```python
from build123d import *

# Parameters (mm, degrees)
CHAMFER1_SIZE = 0.5


with BuildPart() as part:
    # Sketch1 → Revolve1 (revolve)
    with BuildSketch(Plane.XY):
        with BuildLine():
            Line((1.75, 0), (1.75, 10.5))
            Line((1.75, 10.5), (3.9, 10.5))
            Line((3.9, 10.5), (3.9, 5.5))
            Line((3.9, 5.5), (4.9, 5.5))
            ThreePointArc((4.9, 5.5), (5.177696338, 2.695539268), (6, 0))
            Line((6, 0), (1.75, 0))
        make_face()
    revolve(axis=Axis((0, -1052.626814563, 0), (0, 1, 0)))

    # Chamfer1
    # the kernel refuses this chamfer: 0.5 mm, written as the material it takes off along each edge
    with BuildSketch(Plane(origin=(0, 0, 0), x_dir=(1, 0, 0), z_dir=(0, 0, 1))) as chamfer1_piece_1:
        Polygon((1.75 + CHAMFER1_SIZE, 0), (1.75, CHAMFER1_SIZE), (1.75, 0), align=None)
    revolve(axis=Axis((0, 0, 0), (0, 1, 0)), mode=Mode.SUBTRACT)
    with BuildSketch(Plane(origin=(0, 10.5, 0), x_dir=(1, 0, 0), z_dir=(0, 0, 1))) as chamfer1_piece_2:
        Polygon((1.75, -CHAMFER1_SIZE), (1.75 + CHAMFER1_SIZE, 0), (1.75, 0), align=None)
    revolve(axis=Axis((0, 10.5, 0), (0, 1, 0)), mode=Mode.SUBTRACT)
    with BuildSketch(Plane(origin=(0, 10.5, 0), x_dir=(1, 0, 0), z_dir=(0, 0, 1))) as chamfer1_piece_3:
        Polygon((3.9 - CHAMFER1_SIZE, 0), (3.9, -CHAMFER1_SIZE), (3.9, 0), align=None)
    revolve(axis=Axis((0, 10.5, 0), (0, 1, 0)), mode=Mode.SUBTRACT)
    with BuildSketch(Plane(origin=(0, 5.5, 0), x_dir=(1, 0, 0), z_dir=(0, 0, 1))) as chamfer1_piece_4:
        with BuildLine():
            Line((4.9 - CHAMFER1_SIZE, 0), (4.909063924, -0.509063924))
            ThreePointArc((4.909063924, -0.509063924), (4.902396158, -0.261771596), (4.9, 0))
            Line((4.9, 0), (4.9 - CHAMFER1_SIZE, 0))
        make_face()
    revolve(axis=Axis((0, 5.5, 0), (0, 1, 0)), mode=Mode.SUBTRACT)


solid = part.part
```
Read the model definition and answer for the solid it produces. Units are mm, in the model's axes. Coordinates: 2 decimals unless noted, no trailing zeros. Loops run counter-clockwise (first coordinate to the right, second up) from the corner with the lowest first, then second, coordinate; pieces in that order, holes last. Notation, with made-up numbers: (40, -5.75) - (51, -5.75) arc R32 ccw to (51, 24.25) - close; hole circle Ø11 at (55, 21). An arc over 180 degrees is marked (long way). Answer in a Markdown table with one row per item.
1. Determine the mould class of faces 1 (the face through (3, 0, 0)), 2 (the face through (-2.87, 7.72, -2.64)), 3 (the face through (1.617, 5.316, 0.67)) for opening direction X: +X half, -X half, draft (parallel to the pull), parting line (faces both ways), or undercut.
Conclusion:
| item | result |
|---|---|
| face 1 | draft |
| face 2 | parting line |
| face 3 | undercut |
2. Find section A-A, the plane x = 0. Write down the section's boundary in (y, z), then the cut area to 3 significant figures.
Conclusion:
| item | result |
|---|---|
| outline | (0, -6) arc R14.3 cw to (4.99, -4.91) - (5.5, -4.4) - (5.5, -3.9) - (10, -3.9) - (10.5, -3.4) - (10.5, -2.25) - (10, -1.75) - (0.5, -1.75) - (0, -2.25) - close; (0, 2.25) - (0.5, 1.75) - (10, 1.75) - (10.5, 2.25) - (10.5, 3.4) - (10, 3.9) - (5.5, 3.9) - (5.5, 4.4) - (4.99, 4.91) arc R14.3 cw to (0, 6) - close |
| area | 59.1 mm² |
3. Straight lines are drawn through the part: line 1 (Z direction, x = 0, y = 6.5); line 2 (X direction, y = 3, z = -0.5). For each, find the intervals that lie inside material, in ascending order.
Conclusion:
| item | result |
|---|---|
| line 1 | z = -3.9 to -1.75, 1.75 to 3.9 |
| line 2 | x = -5.1 to -1.68, 1.68 to 5.1 |
4. Find section B-B, the plane z = 0. Write down the section's boundary in (x, y), then the cut area to 3 significant figures.
Conclusion:
| item | result |
|---|---|
| outline | (-6, 0) - (-2.25, 0) - (-1.75, 0.5) - (-1.75, 10) - (-2.25, 10.5) - (-3.4, 10.5) - (-3.9, 10) - (-3.9, 5.5) - (-4.4, 5.5) - (-4.91, 4.99) arc R14.3 cw to start; (1.75, 0.5) - (2.25, 0) - (6, 0) arc R14.3 cw to (4.91, 4.99) - (4.4, 5.5) - (3.9, 5.5) - (3.9, 10) - (3.4, 10.5) - (2.25, 10.5) - (1.75, 10) - close |
| area | 59.1 mm² |
5. Given pin 1 (3 mm diameter, centred on x = 0, z = 0, fed in from +Y); pin 2 (4 mm diameter, centred on x = -0.5, z = -0.5, fed in from +Y); pin 3 (2 mm diameter, centred on y = 5.5, z = -3.5, fed in from -X); pin 4 (1.5 mm diameter, centred on y = 3.5, z = 3, fed in from -X), each flat-ended and moving along its own axis, determine where each tip first touches the part or whether it passes through.
Conclusion:
| item | result |
|---|---|
| pin 1 | passes through |
| pin 2 | stops at y = 10.5 |
| pin 3 | stops at x = -4.14 |
| pin 4 | stops at x = -4.53 |
6. Find section D-D, the plane y = 5.25. Write down the section's boundary in (x, z).
Conclusion:
| item | result |
|---|---|
| outline | circle Ø9.3 at (0, 0); hole circle Ø3.5 at (0, 0) |
7. Find section C-C, the plane y = 7.75. Write down the section's boundary in (x, z).
Conclusion:
| item | result |
|---|---|
| outline | circle Ø7.8 at (0, 0); hole circle Ø3.5 at (0, 0) |
